from build123d import *

# Parameters (mm, degrees)
BOSS_EXTRUDE1_DEPTH = 1
SKETCH2_R           = 3.5
CUT_EXTRUDE1_DEPTH  = 24.027157879
SKETCH3_R           = 3
BOSS_EXTRUDE2_DEPTH = 2
CIRPATTERN1_COUNT   = 4
CHAMFER1_SIZE       = 1
CIRPATTERN2_COUNT   = 4
CUT_EXTRUDE4_DEPTH  = 0.25
SKETCH6_R           = 2.5
BOSS_EXTRUDE3_DEPTH = 0.5
CIRPATTERN3_COUNT   = 4
SKETCH7_R           = 0.9
CUT_EXTRUDE5_DEPTH  = 24.092206478


with BuildPart() as part:
    # Sketch1 → Boss-Extrude1 (new body)
    with BuildSketch(Plane(origin=(0, 0, 0), x_dir=(1, 0, 0), z_dir=(0, 1, 0))):
        with BuildLine():
            Line((5, 17), (11.032262936, 10.887569725))
            ThreePointArc((11.032262936, 10.887569725), (15.5, 0), (11.032262936, -10.887569725))
            Line((11.032262936, -10.887569725), (5, -17))
            Line((5, -17), (-5, -17))
            Line((-5, -17), (-11.032262936, -10.887569725))
            ThreePointArc((-11.032262936, -10.887569725), (-15.5, 0), (-11.032262936, 10.887569725))
            Line((-11.032262936, 10.887569725), (-5, 17))
            Line((-5, 17), (5, 17))
        make_face()
    extrude(amount=BOSS_EXTRUDE1_DEPTH)

    # Sketch2 → Cut-Extrude1 (cut, through all)
    with BuildSketch(Plane(origin=(0, 1, 0), x_dir=(1, 0, 0), z_dir=(0, 1, 0))):
        with Locations(Location((0, 0, 0), (0, 0, 270))):
            Circle(SKETCH2_R)
    extrude(amount=-CUT_EXTRUDE1_DEPTH, mode=Mode.SUBTRACT)

    # Sketch3 → Boss-Extrude2 (add)
    with BuildSketch(Plane(origin=(0, 1, 0), x_dir=(1, 0, 0), z_dir=(0, 1, 0))):
        with Locations(Location((-6.363961031, 6.363961031, 0), (0, 0, 270))):
            Circle(SKETCH3_R)
    boss_extrude2 = extrude(amount=BOSS_EXTRUDE2_DEPTH)

    # CirPattern1: Boss-Extrude2 ×4 about axis
    cirpattern1_axis = Axis((0, 0, 0), (0, 1, 0))
    for i in range(1, CIRPATTERN1_COUNT):
        add(boss_extrude2.rotate(cirpattern1_axis, i * 360 / CIRPATTERN1_COUNT))

    # Chamfer1
    chamfer1_edges = [part.edges().sort_by_distance(p)[0] for p in [
        (-6.363961031, 1, -9.363961031),
        (-9.363961031, 1, 6.363961031),
        (6.363961031, 1, 9.363961031),
        (9.363961031, 1, -6.363961031),
    ]]
    chamfer(chamfer1_edges, length=CHAMFER1_SIZE)

    # Sketch4 → Cut-Revolve1 (revolve, cut)
    with BuildSketch(Plane(origin=(0, 0, 0), x_dir=(-0.7071067811865477, 0, -0.7071067811865475), z_dir=(0.7071067811865475, 0, -0.7071067811865477)), mode=Mode.PRIVATE) as cut_revolve1_sk:
        Polygon((12.5, 0), (9, 0), (9, 1.75), (11.5, 1.75), (12.5, 0.5), align=None)
    cut_revolve1 = revolve(cut_revolve1_sk.sketch.rotate(Axis((-6.363961031, 1, -6.363961031), (0, 1, 0)), 315), axis=Axis((-6.363961031, 1, -6.363961031), (0, 1, 0)), mode=Mode.SUBTRACT)

    # CirPattern2: Cut-Revolve1 ×4 about axis
    cirpattern2_axis = Axis((0, 0, 0), (0, 1, 0))
    for i in range(1, CIRPATTERN2_COUNT):
        add(cut_revolve1.rotate(cirpattern2_axis, i * 360 / CIRPATTERN2_COUNT), mode=Mode.SUBTRACT)

    # Sketch5 → Cut-Extrude4 (cut)
    with BuildSketch(Plane.XZ):
        with BuildLine():
            Line((-3.009859064, 7.363961031), (3.009859064, 7.363961031))
            ThreePointArc((3.009859064, 7.363961031), (2.863961031, 6.363961031), (3.009859064, 5.363961031))
            Line((3.009859064, 5.363961031), (-3.009859064, 5.363961031))
            ThreePointArc((-3.009859064, 5.363961031), (-2.863961031, 6.363961031), (-3.009859064, 7.363961031))
        make_face()
        with BuildLine():
            Line((-7.363961031, 3.009859064), (-7.363961031, -3.009859064))
            ThreePointArc((-7.363961031, -3.009859064), (-6.363961031, -2.863961031), (-5.363961031, -3.009859064))
            Line((-5.363961031, -3.009859064), (-5.363961031, 3.009859064))
            ThreePointArc((-5.363961031, 3.009859064), (-6.363961031, 2.863961031), (-7.363961031, 3.009859064))
        make_face()
        with BuildLine():
            Line((-3.009859064, -5.363961031), (3.009859064, -5.363961031))
            ThreePointArc((3.009859064, -5.363961031), (2.863961031, -6.363961031), (3.009859064, -7.363961031))
            Line((3.009859064, -7.363961031), (-3.009859064, -7.363961031))
            ThreePointArc((-3.009859064, -7.363961031), (-2.863961031, -6.363961031), (-3.009859064, -5.363961031))
        make_face()
        with BuildLine():
            Line((5.363961031, -3.009859064), (5.363961031, 3.009859064))
            ThreePointArc((5.363961031, 3.009859064), (6.363961031, 2.863961031), (7.363961031, 3.009859064))
            Line((7.363961031, 3.009859064), (7.363961031, -3.009859064))
            ThreePointArc((7.363961031, -3.009859064), (6.363961031, -2.863961031), (5.363961031, -3.009859064))
        make_face()
        with BuildLine():
            Line((8.028562495, 9.442776057), (10.257954735, 11.672168297))
            Line((10.257954735, 11.672168297), (11.032262936, 10.887569725))
            ThreePointArc((11.032262936, 10.887569725), (11.343108447, 10.563327637), (11.644428208, 10.230214646))
            Line((11.644428208, 10.230214646), (9.442776057, 8.028562495))
            ThreePointArc((9.442776057, 8.028562495), (8.838834765, 8.838834765), (8.028562495, 9.442776057))
        make_face()
        with BuildLine():
            Line((-8.028562495, 9.442776057), (-10.257954735, 11.672168297))
            Line((-10.257954735, 11.672168297), (-11.032262936, 10.887569725))
            ThreePointArc((-11.032262936, 10.887569725), (-11.343108447, 10.563327637), (-11.644428208, 10.230214646))
            Line((-11.644428208, 10.230214646), (-9.442776057, 8.028562495))
            ThreePointArc((-9.442776057, 8.028562495), (-8.838834765, 8.838834765), (-8.028562495, 9.442776057))
        make_face()
        with BuildLine():
            Line((-8.028562495, -9.442776057), (-10.257954735, -11.672168297))
            Line((-10.257954735, -11.672168297), (-11.032262936, -10.887569725))
            ThreePointArc((-11.032262936, -10.887569725), (-11.343108447, -10.563327637), (-11.644428208, -10.230214646))
            Line((-11.644428208, -10.230214646), (-9.442776057, -8.028562495))
            ThreePointArc((-9.442776057, -8.028562495), (-8.838834765, -8.838834765), (-8.028562495, -9.442776057))
        make_face()
        with BuildLine():
            Line((8.028562495, -9.442776057), (10.257954735, -11.672168297))
            Line((10.257954735, -11.672168297), (11.032262936, -10.887569725))
            ThreePointArc((11.032262936, -10.887569725), (11.343108447, -10.563327637), (11.644428208, -10.230214646))
            Line((11.644428208, -10.230214646), (9.442776057, -8.028562495))
            ThreePointArc((9.442776057, -8.028562495), (8.838834765, -8.838834765), (8.028562495, -9.442776057))
        make_face()
    extrude(amount=-CUT_EXTRUDE4_DEPTH, mode=Mode.SUBTRACT)

    # Sketch6 → Boss-Extrude3 (add)
    with BuildSketch(Plane.XZ.offset(-1.75)):
        with Locations(Location((-6.363961031, -6.363961031, 0), (0, 0, 270))):
            Circle(SKETCH6_R)
    boss_extrude3 = extrude(amount=BOSS_EXTRUDE3_DEPTH)

    # CirPattern3: Boss-Extrude3 ×4 about axis
    cirpattern3_axis = Axis((0, 0, 0), (0, 1, 0))
    for i in range(1, CIRPATTERN3_COUNT):
        add(boss_extrude3.rotate(cirpattern3_axis, i * 360 / CIRPATTERN3_COUNT))

    # Sketch7 → Cut-Extrude5 (cut, through all)
    with BuildSketch(Plane(origin=(0, 1, 0), x_dir=(1, 0, 0), z_dir=(0, 1, 0))):
        with Locations(Location((0, 15, 0), (0, 0, 270))):
            Circle(SKETCH7_R)
    cut_extrude5 = extrude(amount=-CUT_EXTRUDE5_DEPTH, mode=Mode.SUBTRACT)

    # Mirror1: Cut-Extrude5 across plane
    add(cut_extrude5.mirror(Plane.XY), mode=Mode.SUBTRACT)


solid = part.part
Work out the finished part from the listing and answer in its coordinate system (mm). A direction names the side the tool comes from. Round coordinates to 2 decimals unless told otherwise and drop trailing zeros. Order: outer loops, then holes, each group sorted by start corner. A loop starts at its lowest first (then second) coordinate and runs counter-clockwise, first axis right, second up. Notation, with made-up numbers: M 39,-1 L 97,-1 A26 ccw 97,37 Z; hole C 13.5,-6.5 d4. An arc over 180 degrees is marked long. One line per item, written item: value.
Q1. For faces 5 (the face through (0.27, 0.51, 14.14)), 6 (the face through (10, 0.25, 10)), determine the directions among +Z, -Z, +X, -X, +Y, -Y from which every point of the face is accessible in a straight line to the end or side of a thin tool.
Derived:
face 5: +Y, -Y
face 6: -Y
Q2. Find section C-C on y = 2.55. Write down the section's boundary in (x, z), then the cut area to 3 significant figures.
Derived:
outline: C -6.36,-6.36 d6; C -6.36,6.36 d6; C 6.36,-6.36 d6; C 6.36,6.36 d6
area: 113 mm²
Q3. Flat-ended cylindrical pins translate along their axes: pin 1 (1.6 mm diameter, centred on x = -6.5, z = -1.5, fed in from -Y); pin 2 (6.5 mm diameter, centred on x = 6.36, z = 6.36, fed in from -Y); pin 3 (5 mm diameter, centred on x = -11.5, z = 11.5, fed in from +Y); pin 4 (1.1 mm diameter, centred on x = 0, z = 15, fed in from +Y). Find the tip coordinate at first contact, or state that the pin passes through.
Derived:
pin 1: y = 0.25
pin 2: y = 0.81
pin 3: y = 1
pin 4: through
Q4. Find section A-A on z = 0. Write down the section's boundary in (x, y), then the cut area to 3 significant figures.
Derived:
outline: M -15.5,0 L -7.36,0 L -7.36,0.25 L -5.36,0.25 L -5.36,0 L -3.5,0 L -3.5,1 L -15.5,1 Z; M 3.5,0 L 5.36,0 L 5.36,0.25 L 7.36,0.25 L 7.36,0 L 15.5,0 L 15.5,1 L 3.5,1 Z
area: 23.0 mm²
Q5. Find section D-D on z = -15. Write down the section's boundary in (x, y).
Derived:
outline: M -6.97,0 L -0.9,0 L -0.9,1 L -6.97,1 Z; M 0.9,0 L 6.97,0 L 6.97,1 L 0.9,1 Z
Q6. Straight lines are drawn through the part: line 1 (X direction, y = 0.2, z = 0); line 2 (X direction, y = 0.8, z = -5.5); line 3 (Z direction, x = 8.5, y = 1.1). For each, find the intervals that lie inside material, in ascending order.
Derived:
line 1: -15.5 to -7.36, -5.36 to -3.5, 3.5 to 5.36, 7.36 to 15.5
line 2: -14.49 to -9.51, -3.22 to 3.22, 9.51 to 14.49
line 3: -9.63 to -8.5, -4.23 to -3.1, 3.1 to 4.23, 8.5 to 9.63
Q7. Determine the mould class of faces 1 (the face through (8.06, 0.49, 13.9)), 2 (the face through (-6, 3, 6)), 3 (the face through (-15.5, 0.5, 0.2)), 4 (the face through (-7.42, 0.25, -9.7)) for opening direction X: released by +X, released by -X, zero draft, split by the parting line, or undercut.
Derived:
face 1: released by +X
face 2: zero draft
face 3: released by -X
face 4: undercut
Q8. Find section B-B on x = 0. Write down the section's boundary in (y, z), then the cut area to 3 significant figures.
Derived:
outline: M 0,-17 L 1,-17 L 1,-15.9 L 0,-15.9 Z; M 0,-14.1 L 1,-14.1 L 1,-3.5 L 0,-3.5 L 0,-5.36 L 0.25,-5.36 L 0.25,-7.36 L 0,-7.36 Z; M 0,3.5 L 1,3.5 L 1,14.1 L 0,14.1 L 0,7.36 L 0.25,7.36 L 0.25,5.36 L 0,5.36 Z; M 0,15.9 L 1,15.9 L 1,17 L 0,17 Z
area: 22.4 mm²
